Part model, mm, in its own coordinate system. A direction names the side the tool comes from. Round coordinates to 2 decimals unless told otherwise and drop trailing zeros. Loops run counter-clockwise (first coordinate to the right, second up) from the corner with the lowest first, then second, coordinate; pieces in that order, holes last. Notation, with made-up numbers: M -20,8.5 L 28,8.5 A12 cw 28,13.5 Z; hole C 69.5,20 d7. An arc over 180 degrees is marked long. Answer as CSV lines item,"result". Start each with the question number.
Item 1: Which spindle directions (+Z, -Z, +X, -X, +Y, -Y) get a long thin tool onto all of the face, cutting with end or side? Do faces 4 (the flat face through (14, 11, 8)), 5 (the cylindrical face through (29, 3, 22)), 6 (the flat face through (-26.5, -7, 33)), 7 (the flat face through (6, 11, 32)), 8 (the cylindrical face through (19.5, -0.1, 1.5)). Say none if no direction does.
Item 2: Mould opens along X. For faces 1 (the flat face through (0, -17.5, 22)), 2 (the flat face through (-25.98, -10.8, 44.51)), 3 (the flat face through (-13.606, 14.87, 26.759)) say: pulls with the +X half, pulls with the -X half, needs draft (parallel to the pull), parting line crosses it, or undercut.
Item 3: Wall check: line 1 (Z direction, x = -14, y = -6); line 2 (X direction, y = 12, z = 18.5); line 3 (Y direction, x = 15, z = 2.5). Give the ranges that are in metal, low to high.
Item 4: Band-saw the part on A-A (x = -22.5). Give the cut face in (y, z), and give its area (3 significant figures).
Item 5: Drop flat-ended pins along their axis: pin 1 Ø3.5 at (y, z) = (13, 21.5) entering from -X; pin 2 Ø2 at (x, y) = (-3, 5.5) entering from -Z; pin 3 Ø5 at (y, z) = (6, 22) entering from +X. Give the stop position or say it passes through.
```python
from build123d import *

# Parameters (mm, degrees)
SKETCH_R             = 1.6
PAD_DEPTH            = 45
SKETCH001_R          = 4.1
POCKET_DEPTH         = 37
SKETCH002_R          = 9.6
POCKET001_DEPTH      = 17.501
POCKET001_DEPTH_BACK = 17.501
SKETCH003_R          = 2.5
SKETCH003_W          = 35
SKETCH003_H          = 6
POCKET002_DEPTH      = 5.5
SKETCH004_R          = 4
POCKET003_DEPTH      = 5
SKETCH005_R          = 2.5
POCKET004_DEPTH      = 5.5
SKETCH006_R          = 4
POCKET005_DEPTH      = 5
SKETCH007_R          = 1.25
POCKET006_DEPTH      = 32.501
POCKET006_DEPTH_BACK = 32.501
SKETCH008_R          = 1.6
POCKET007_DEPTH      = 20
SKETCH009_R          = 3
POCKET008_DEPTH      = 6
SKETCH010_R          = 3
POCKET009_DEPTH      = 6
SKETCH011_R          = 3
POCKET010_DEPTH      = 3
CHAMFER_SIZE         = 1
CHAMFER001_SIZE      = 0.4


with BuildPart() as part:
    # Sketch → Pad (new body)
    with BuildSketch(Plane.XY):
        Polygon((-32.5, 5), (-32.5, -5), (-20, -17.5), (20, -17.5), (32.5, -5), (32.5, 5), (20, 17.5), (-20, 17.5), align=None)
        with Locations((-15, 12.5)):
            Circle(SKETCH_R, mode=Mode.SUBTRACT)
        with Locations((-15, -12.5)):
            Circle(SKETCH_R, mode=Mode.SUBTRACT)
        with Locations((15, -12.5)):
            Circle(SKETCH_R, mode=Mode.SUBTRACT)
        with Locations((15, 12.5)):
            Circle(SKETCH_R, mode=Mode.SUBTRACT)
        with Locations((22.5, 0)):
            Circle(SKETCH_R, mode=Mode.SUBTRACT)
        with Locations((-22.5, 0)):
            Circle(SKETCH_R, mode=Mode.SUBTRACT)
    extrude(amount=PAD_DEPTH)

    # Sketch001 (on Face16 of Pad) → Pocket (cut)
    with BuildSketch(Plane.XY.offset(45)):
        with Locations((-22.5, 0)):
            Circle(SKETCH001_R)
        with Locations((22.5, 0)):
            Circle(SKETCH001_R)
        Polygon((-12.25, 10.912287), (-12.25, 14.087713), (-15, 15.675426), (-17.75, 14.087713), (-17.75, 10.912287), (-15, 9.324574), align=None)
        Polygon((17.75, 10.912287), (17.75, 14.087713), (15, 15.675426), (12.25, 14.087713), (12.25, 10.912287), (15, 9.324574), align=None)
        Polygon((-12.25, -14.087713), (-12.25, -10.912287), (-15, -9.324574), (-17.75, -10.912287), (-17.75, -14.087713), (-15, -15.675426), align=None)
        Polygon((17.75, -14.087713), (17.75, -10.912287), (15, -9.324574), (12.25, -10.912287), (12.25, -14.087713), (15, -15.675426), align=None)
    extrude(amount=-POCKET_DEPTH, mode=Mode.SUBTRACT)

    # Sketch002 → Pocket001 (cut, two sides)
    with BuildSketch(Plane.XZ) as pocket001_sk:
        Circle(SKETCH002_R)
    extrude(amount=-POCKET001_DEPTH, mode=Mode.SUBTRACT)
    extrude(pocket001_sk.sketch, amount=POCKET001_DEPTH_BACK, mode=Mode.SUBTRACT)

    # Sketch003 (on DatumPlane) → Pocket002 (cut, symmetric)
    with BuildSketch(Plane.YZ.offset(-6)):
        with BuildLine():
            ThreePointArc((-6, 24), (1.071068, 26.928932), (4, 34))
            Line((4, 45), (4, 34))
            Line((-17.5, 45), (4, 45))
            Line((-17.5, 24), (-17.5, 45))
            Line((-6, 24), (-17.5, 24))
        make_face()
        with Locations((-6, 34)):
            Circle(SKETCH003_R, mode=Mode.SUBTRACT)
        with Locations((0, 15)):
            Rectangle(SKETCH003_W, SKETCH003_H)
    extrude(amount=POCKET002_DEPTH, both=True, mode=Mode.SUBTRACT)

    # Sketch004 (on DatumPlane) → Pocket003 (cut, symmetric)
    with BuildSketch(Plane.YZ.offset(-6)):
        with Locations((-6, 34)):
            Circle(SKETCH004_R)
    extrude(amount=POCKET003_DEPTH, both=True, mode=Mode.SUBTRACT)

    # Sketch005 (on DatumPlane) → Pocket004 (cut, symmetric)
    with BuildSketch(Plane.YZ.offset(6)):
        with BuildLine():
            ThreePointArc((-4, 22), (-1.071068, 14.928932), (6, 12))
            Line((17.5, 12), (6, 12))
            Line((17.5, 32), (17.5, 12))
            Line((4, 32), (17.5, 32))
            Line((4, 45), (4, 32))
            Line((-4, 45), (4, 45))
            Line((-4, 22), (-4, 45))
        make_face()
        with Locations((6, 22)):
            Circle(SKETCH005_R, mode=Mode.SUBTRACT)
    extrude(amount=POCKET004_DEPTH, both=True, mode=Mode.SUBTRACT)

    # Sketch006 (on DatumPlane) → Pocket005 (cut, symmetric)
    with BuildSketch(Plane.YZ.offset(6)):
        with Locations((6, 22)):
            Circle(SKETCH006_R)
    extrude(amount=POCKET005_DEPTH, both=True, mode=Mode.SUBTRACT)

    # Sketch007 → Pocket006 (cut, two sides)
    with BuildSketch(Plane.YZ) as pocket006_sk:
        with Locations((-6, 34)):
            Circle(SKETCH007_R)
        with Locations((6, 22)):
            Circle(SKETCH007_R)
    extrude(amount=-POCKET006_DEPTH, mode=Mode.SUBTRACT)
    extrude(pocket006_sk.sketch, amount=POCKET006_DEPTH_BACK, mode=Mode.SUBTRACT)

    # Sketch008 → Pocket007 (cut, symmetric)
    with BuildSketch(Plane.YZ):
        with Locations((-6, 34)):
            Circle(SKETCH008_R)
        with Locations((6, 22)):
            Circle(SKETCH008_R)
    extrude(amount=POCKET007_DEPTH, both=True, mode=Mode.SUBTRACT)

    # Sketch009 (on Face16 of Pocket007) → Pocket008 (cut)
    with BuildSketch(Plane.YZ.offset(32.5)):
        with Locations((6, 22)):
            Circle(SKETCH009_R)
    extrude(amount=-POCKET008_DEPTH, mode=Mode.SUBTRACT)

    # Sketch010 (on Face1 of Pocket008) → Pocket009 (cut)
    with BuildSketch(Plane(origin=(-32.5, 0, 0), x_dir=(0, -1, 0), z_dir=(-1, 0, 0))):
        with Locations((6, 34)):
            Circle(SKETCH010_R)
    extrude(amount=-POCKET009_DEPTH, mode=Mode.SUBTRACT)

    # Sketch011 (on Face2 of Pocket009) → Pocket010 (cut)
    with BuildSketch(Plane(origin=(0, 0, 0), x_dir=(1, 0, 0), z_dir=(0, 0, -1))):
        with Locations((-22.5, 0)):
            Circle(SKETCH011_R)
        with Locations((22.5, 0)):
            Circle(SKETCH011_R)
    extrude(amount=-POCKET010_DEPTH, mode=Mode.SUBTRACT)

    # Chamfer
    chamfer_edges = [part.edges().sort_by_distance(p)[0] for p in [
        (-15.75, -17.5, 45),
        (-26.25, -11.25, 45),
        (-32.5, 0, 45),
        (-26.25, 11.25, 45),
        (0, 17.5, 45),
        (26.25, 11.25, 45),
        (32.5, 0, 45),
        (26.25, -11.25, 45),
        (9.75, -17.5, 45),
    ]]
    chamfer(chamfer_edges, length=CHAMFER_SIZE)

    # Chamfer001
    chamfer001_edges = [part.edges().sort_by_distance(p)[0] for p in [
        (-11, -8.5, 34),
        (-1, -8.5, 34),
        (1, 3.5, 22),
        (11, 3.5, 22),
    ]]
    chamfer(chamfer001_edges, length=CHAMFER001_SIZE)


solid = part.part
```
Answer block:
1,face 4,"+Z"
1,face 5,"+X"
1,face 6,"-X"
1,face 7,"+Y"
1,face 8,"-Z"
2,face 1,"needs draft"
2,face 2,"pulls with the -X half"
2,face 3,"undercut"
3,line 1,"z = 0 to 32.4, 35.6 to 45"
3,line 2,"x = -25.5 to -17.75, -12.25 to 0.5, 11.5 to 12.25, 17.75 to 25.5"
3,line 3,"y = -17.5 to -14.1, -10.9 to 10.9, 14.1 to 17.5"
4,outline,"M -15,0 L -3,0 L -3,3 L -1.6,3 L -1.6,8 L -4.1,8 L -4.1,45 L -13.59,45 L -15,44 Z; M 1.6,3 L 3,3 L 3,0 L 15,0 L 15,44 L 13.59,45 L 4.1,45 L 4.1,8 L 1.6,8 Z; hole C -6,34 d2.5; hole C 6,22 d2.5"
4,area,"1,000 mm^2"
5,pin 1,"stops at x = -26.25"
5,pin 2,"stops at z = 8.73"
5,pin 3,"stops at x = 26.5"
